Can you work these out from the model? Positions are in its coordinate system, mm. A direction names the side the tool comes from. Round coordinates to 2 decimals unless told otherwise and drop trailing zeros. Answer as CSV lines item,"result".
from build123d import *

# Parameters (mm, degrees)
PAD_DEPTH       = 155
SKETCH001_W     = 15
SKETCH001_H     = 92
SKETCH001_R     = 2.25
PAD001_DEPTH    = 15
POCKET_DEPTH    = 132
FILLET_R        = 10
CHAMFER_SIZE    = 9.99999
FILLET001_R     = 19.9
SKETCH004_W     = 50
SKETCH004_H     = 85
POCKET001_DEPTH = 5
CHAMFER001_SIZE = 3
SKETCH005_R     = 2.1
POCKET002_DEPTH = 92.001
CHAMFER002_SIZE = 1
CHAMFER003_SIZE = 1
CHAMFER004_SIZE = 1


with BuildPart() as part:
    # Sketch → Pad (new body)
    with BuildSketch(Plane.XZ):
        Polygon((40, 0), (40, 17), (0, 17), (0, 92), (-22, 92), (-22, 0), align=None)
    extrude(amount=-PAD_DEPTH)

    # Sketch001 → Pad001 (join)
    with BuildSketch(Plane.XZ):
        with Locations((-29.5, 46)):
            Rectangle(SKETCH001_W, SKETCH001_H)
        with Locations((-27, 77)):
            Circle(SKETCH001_R, mode=Mode.SUBTRACT)
        with Locations((-27, 15)):
            Circle(SKETCH001_R, mode=Mode.SUBTRACT)
    extrude(amount=-PAD001_DEPTH)

    # Sketch002 (on Face5 of Pad001) → Pocket (cut)
    with BuildSketch(Plane(origin=(0, 147, 0), x_dir=(-1, 0, 0), z_dir=(0, 1, 0))):
        Polygon((-40, 0), (-40, 10), (12, 10), (12, 84), (22, 84), (22, 0), align=None)
    extrude(amount=-POCKET_DEPTH, mode=Mode.SUBTRACT)

    # Fillet
    fillet_edges = [part.edges().sort_by_distance(p)[0] for p in [
        (-37, 7.5, 0),
        (-37, 7.5, 92),
        (-12, 81, 10),
    ]]
    fillet(fillet_edges, radius=FILLET_R)

    # Chamfer
    chamfer_edges = [part.edges().sort_by_distance(p)[0] for p in [
        (-12, 81, 84),
        (-12, 147, 52),
    ]]
    chamfer(chamfer_edges, length=CHAMFER_SIZE)

    # Fillet001
    fillet001_edges = [part.edges().sort_by_distance(p)[0] for p in [
        (-22, 151, 0),
    ]]
    fillet(fillet001_edges, radius=FILLET001_R)

    # Sketch004 (on Face5 of Fillet001) → Pocket001 (cut)
    with BuildSketch(Plane(origin=(0, 155, 0), x_dir=(-1, 0, 0), z_dir=(0, 1, 0))):
        with Locations((-15, 49.5)):
            Rectangle(SKETCH004_W, SKETCH004_H)
    extrude(amount=-POCKET001_DEPTH, mode=Mode.SUBTRACT)

    # Chamfer001
    chamfer001_edges = [part.edges().sort_by_distance(p)[0] for p in [
        (19, 15, 10),
    ]]
    chamfer(chamfer001_edges, length=CHAMFER001_SIZE)

    # Sketch005 → Pocket002 (cut, through all)
    with BuildSketch(Plane.XY):
        with Locations((20, 25)):
            Circle(SKETCH005_R)
        with Locations((20, 125)):
            Circle(SKETCH005_R)
    extrude(amount=POCKET002_DEPTH, mode=Mode.SUBTRACT)

    # Chamfer002
    chamfer002_edges = [part.edges().sort_by_distance(p)[0] for p in [
        (17.9, 25, 17),
        (17.9, 125, 17),
        (17.9, 125, 10),
        (17.9, 25, 10),
    ]]
    chamfer(chamfer002_edges, length=CHAMFER002_SIZE)

    # Chamfer003
    chamfer003_edges = [part.edges().sort_by_distance(p)[0] for p in [
        (-13.5, 0, 92),
        (-34.071068, 0, 89.071068),
        (0, 0, 54.5),
        (-37, 0, 46),
        (20, 0, 17),
        (-34.071068, 0, 2.928932),
        (40, 0, 8.5),
        (6.5, 0, 0),
        (-29.25, 0, 15),
        (-29.25, 0, 77),
    ]]
    chamfer(chamfer003_edges, length=CHAMFER003_SIZE)

    # Chamfer004
    chamfer004_edges = [part.edges().sort_by_distance(p)[0] for p in [
        (6.5, 15, 0),
        (-29.25, 15, 77),
        (-29.25, 15, 15),
    ]]
    chamfer(chamfer004_edges, length=CHAMFER004_SIZE)


solid = part.part
Item 1: If we section it at B-B on x = 20: State how many separate pieces and enclosed holes the cut face has, then the cut area to 3 significant figures.
Output:
separate pieces,"3"
enclosed holes,"0"
area,"1,260 mm2"
Item 2: On a 3-axis mill with a long thin cutter (end or side, diameter ignored), from which of +Z, -Z, +X, -X, +Y, -Y can I reach the whole of each face in a straight line? I mean faces 5 (the face through (20, 74, 17)), 6 (the face through (19, 78, 10)), 7 (the face through (-9.15, 76.67, 13.01)). Say none if no direction works.
Output:
face 5,"+Z, +X, +Y, -Y"
face 6,"-Z, +X, -X"
face 7,"-Z, -X"
Item 3: If I drill on line 1 along Y through (x, z) = (20, 13); line 2 along Z through (x, y) = (-27, 4); line 3 along Z through (x, y) = (6, 66), over which ranges is the centre line in solid material (lowest first)? Write a range as from..to.
Output:
line 1,"y = 0..22.9, 27.1..122.9, 127.1..150"
line 2,"z = 0..12.75, 17.25..74.75, 79.25..92"
line 3,"z = 10..17"
Item 4: Will these pins go through, and if not, where does the flat tip stop? pin 1 (5.5 mm diameter, centred on x = 16, y = 153.5, fed in from +Z); pin 2 (15 mm diameter, centred on x = 8.5, z = 47.5, fed in from +Y); pin 3 (2.5 mm diameter, centred on y = 153, z = 70, fed in from +X); pin 4 (5.5 mm diameter, centred on x = 20, y = 125, fed in from +Z).
Output:
pin 1,"stops at z = 7"
pin 2,"passes through"
pin 3,"stops at x = -10"
pin 4,"stops at z = 16.65"
Item 5: We'd pull the mould along X, two halves only. Please class faces 1 (the face through (-25.962, 7.409, 13.004)), 2 (the face through (-22, 100, 85)), 3 (the face through (-11, 77, 92)), 4 (the face through (40, 77, 12)): released by +X, released by -X, zero draft, split by the parting line, or undercut.
Output:
face 1,"undercut"
face 2,"released by -X"
face 3,"zero draft"
face 4,"released by +X"
